Source: CAD feature listing. Evaluate the final solid. Frame: model axes, mm. A direction names the side the tool comes from. Coordinates: 2 decimals unless noted, no trailing zeros. Write each loop counter-clockwise with the first axis right and the second up, starting at its lowest first coordinate (ties: lowest second). Pieces come first, ordered by that corner, then holes. Notation, with made-up numbers: (67.25, 21) - (103.25, 21) arc R27 ccw to (103.25, 39) - close; hole circle Ø8 at (46, 54.25). An arc over 180 degrees is marked (long way). One line per question, with ' | ' between items.
from build123d import *

# Parameters (mm, degrees)
SKETCH1_W                      = 81.28
SKETCH1_H                      = 12.6365
CHAMFER1_SIZE                  = 0.635
LPATTERN3_COUNT                = 2
LPATTERN3_PITCH                = 41.275
F_8_32_TAPPED_HOLE1_AT_2_COUNT = 2
F_8_32_TAPPED_HOLE1_AT_2_PITCH = 15.875


with BuildPart() as part:
    # Sketch1 → Base-Revolve (revolve)
    with BuildSketch(Plane(origin=(0, 0, 0), x_dir=(0, 0, -1), z_dir=(1, 0, 0)), mode=Mode.PRIVATE) as base_revolve_sk:
        with Locations((0, 6.31825)):
            Rectangle(SKETCH1_W, SKETCH1_H)
    revolve(base_revolve_sk.sketch.rotate(Axis((0, 0, 40.64), (0, 0, -1)), 90), axis=Axis((0, 0, 40.64), (0, 0, -1)))  # turned: the seam where the file's is

    # Chamfer1
    chamfer1_edges = [part.edges().sort_by_distance(p)[0] for p in [
        (-12.6365, 0, -40.64),
        (-12.6365, 0, 40.64),
    ]]
    chamfer(chamfer1_edges, length=CHAMFER1_SIZE)

    # Sketch17 → 1_2-13 Tapped Hole1 (revolve, cut)
    with BuildSketch(Plane(origin=(0, 12.6365, -20.6375), x_dir=(0, 0, 1), z_dir=(1, 0, 0))):
        Polygon((0, 0), (0, 25.273), (10.541, 25.273), (6.35, 22.853325022), (6.35, 2.419674978), (10.541, 0), align=None)
    f_1_2_13_tapped_hole1 = revolve(axis=Axis((0, 18.9865, -20.6375), (0, -1, 0)), mode=Mode.SUBTRACT)

    # LPattern3: 1_2-13 Tapped Hole1 ×2
    with Locations(*[(0, 0, i * LPATTERN3_PITCH) for i in range(1, LPATTERN3_COUNT)]):
        add(f_1_2_13_tapped_hole1, mode=Mode.SUBTRACT)

    # Sketch19 → 8-32 Tapped Hole1 (revolve, cut)
    with BuildSketch(Plane(origin=(7.9375, 0, 40.64), x_dir=(0, -1, 0), z_dir=(1, 0, 0))):
        Polygon((0, 0), (0, 9.927806461), (1.7272, 8.89), (1.7272, 5.08), (2.0828, 5.08), (2.0828, 0.190641059), (2.413, 0), align=None)
    f_8_32_tapped_hole1 = revolve(axis=Axis((7.9375, 0, 46.99), (0, 0, -1)), mode=Mode.SUBTRACT)

    # 8-32 Tapped Hole1 at 2: 8-32 Tapped Hole1 ×2
    with Locations(*[(-i * F_8_32_TAPPED_HOLE1_AT_2_PITCH, 0, 0) for i in range(1, F_8_32_TAPPED_HOLE1_AT_2_COUNT)]):
        add(f_8_32_tapped_hole1, mode=Mode.SUBTRACT)

    # Mirror1: 8-32 Tapped Hole1 across plane
    add(f_8_32_tapped_hole1.mirror(Plane.XY), mode=Mode.SUBTRACT)

    # Mirror1 copy 1 sketch → Mirror1 copy 1 (revolve, cut)
    with BuildSketch(Plane(origin=(-7.9375, 0, -40.64), x_dir=(0, -1, 0), z_dir=(1, 0, 0))):
        Polygon((0, 0), (0, -9.927806461), (1.7272, -8.89), (1.7272, -5.08), (2.0828, -5.08), (2.0828, -0.190641059), (2.413, 0), align=None)
    revolve(axis=Axis((-7.9375, 0, -46.99), (0, 0, -1)), mode=Mode.SUBTRACT)


solid = part.part
Item 1: Cut plane B-B on y = 11. State how many separate pieces and enclosed holes the cut face has, and give its area (3 significant figures).
Check sheet entries:
separate pieces: 3 | enclosed holes: 0 | area: 673 mm²
Item 2: Cut plane A-A on x = 0. Return loops of the section in (y, z) (1 decimal), and give its area (3 significant figures).
Check sheet entries:
outline: (-12.6, -40) - (-12, -40.6) - (12, -40.6) - (12.6, -40) - (12.6, -31.2) - (10.2, -27) - (-10.2, -27) - (-12.6, -31.2) - close; (-12.6, -10.1) - (-10.2, -14.3) - (10.2, -14.3) - (12.6, -10.1) - (12.6, 10.1) - (10.2, 14.3) - (-10.2, 14.3) - (-12.6, 10.1) - close; (-12.6, 31.2) - (-10.2, 27) - (10.2, 27) - (12.6, 31.2) - (12.6, 40) - (12, 40.6) - (-12, 40.6) - (-12.6, 40) - close | area: 1,370 mm²
Item 3: Pin query (flat end, axial travel): pin 1 Ø3 at (x, y) = (-7.94, 0) entering from -Z (3 decimals); pin 2 Ø2 at (x, y) = (-7.5, -0.5) entering from -Z; pin 3 Ø3 at (x, y) = (7.94, 0) entering from +Z (3 decimals); pin 4 Ø2 at (x, z) = (-0.5, 16) entering from -Y. Return the tip coordinate at first contact, or that it passes through.
Check sheet entries:
pin 1: z = -31.615 | pin 2: z = -31.71 | pin 3: z = 31.615 | pin 4: through
Item 4: Cut plane C-C on z = 34.5. Return loops of the section in (x, y), and give its area (3 significant figures).
Check sheet entries:
outline: circle Ø25.27 at (0, 0); hole circle Ø3.45 at (-7.94, 0); hole circle Ø3.45 at (7.94, 0) | area: 483 mm²
Item 5: Mould query, pull axis X, two halves, no side actions, for faces 4 (the face through (0, 0, -40.64)), 5 (the face through (8.23, 0.065, -30.892)). Classes: pulls with the +X half, pulls with the -X half, needs draft (parallel to the pull), parting line crosses it, or undercut.
Check sheet entries:
face 4: needs draft | face 5: undercut
Item 6: Access query for faces 1 (the face through (9.97, 0.45, -38.04)), 2 (the face through (5.81, -10.33, 23.66)), 3 (the face through (6.225, 0.225, 33.682)). Directions: +Z, -Z, +X, -X, +Y, -Y. A direction counts if a zero-diameter tool reaches every point of the face in a straight line with its end or side. Return the directions, or none.
Check sheet entries:
face 1: -Z | face 2: -Y | face 3: +Z
Item 7: Cut plane D-D on z = -1. Return loops of the section in (x, y), and give its area (3 significant figures).
Check sheet entries:
outline: circle Ø25.27 at (0, 0) | area: 502 mm²
Item 8: Ray query, line 1 along Z through (x, y) = (0, 2.25); line 2 along Z through (x, y) = (-1, 9.25); line 3 along Y through (x, z) = (6.25, -37). Return the intervals inside material, ascending. Write a range as [from, to].
Check sheet entries:
line 1: [-40.64, -26.99], [-14.29, 14.29], [26.99, 40.64] | line 2: [-40.64, -26.91], [-14.37, 14.37], [26.91, 40.64] | line 3: [-10.98, -1.22], [1.22, 10.98]
